```python
from build123d import *

# Parameters (mm, degrees)
SKETCH1_W           = 45
SKETCH1_H           = 57
BOSS_EXTRUDE1_DEPTH = 10
SKETCH4_W           = 45
SKETCH4_H           = 10
BOSS_EXTRUDE4_DEPTH = 35
SKETCH5_W           = 5
SKETCH5_H           = 20
SKETCH5_W_2         = 2
BOSS_EXTRUDE5_DEPTH = 45
CUT_EXTRUDE1_START  = -30
SKETCH6_R           = 1.75
CUT_EXTRUDE1_DEPTH  = 30


with BuildPart() as part:
    # Sketch1 → Boss-Extrude1 (new body)
    with BuildSketch(Plane(origin=(0, 0, 0), x_dir=(1, 0, 0), z_dir=(0, 1, 0))):
        Rectangle(SKETCH1_W, SKETCH1_H)
        with BuildLine():
            ThreePointArc((-15, -19.5), (-18, -16.5), (-15, -13.5))
            Line((-15, -13.5), (15, -13.5))
            ThreePointArc((15, -13.5), (17.121320344, -14.378679656), (18, -16.5))
            ThreePointArc((18, -16.5), (17.121320344, -18.621320344), (15, -19.5))
            Line((15, -19.5), (-15, -19.5))
        make_face(mode=Mode.SUBTRACT)
    extrude(amount=BOSS_EXTRUDE1_DEPTH)

    # Sketch4 → Boss-Extrude4 (add)
    with BuildSketch(Plane(origin=(0, 0, -28.5), x_dir=(-1, 0, 0), z_dir=(0, 0, -1))):
        with Locations((0, 5)):
            Rectangle(SKETCH4_W, SKETCH4_H)
    extrude(amount=BOSS_EXTRUDE4_DEPTH)

    # Sketch5 → Boss-Extrude5 (add)
    with BuildSketch(Plane(origin=(22.5, 0, 0), x_dir=(0, 0, -1), z_dir=(1, 0, 0))):
        with Locations((36, 20)):
            Rectangle(SKETCH5_W, SKETCH5_H)
        with Locations((48.5, 20)):
            Rectangle(SKETCH5_W_2, SKETCH5_H)
        with Locations((61, 20)):
            Rectangle(SKETCH5_W, SKETCH5_H)
    extrude(amount=-BOSS_EXTRUDE5_DEPTH)

    # Sketch6 → Cut-Extrude1 (cut)
    with BuildSketch(Plane.XY.offset(-33.5).offset(CUT_EXTRUDE1_START)):
        with Locations((0, 20)):
            Circle(SKETCH6_R)
    extrude(amount=CUT_EXTRUDE1_DEPTH, mode=Mode.SUBTRACT)


solid = part.part
```
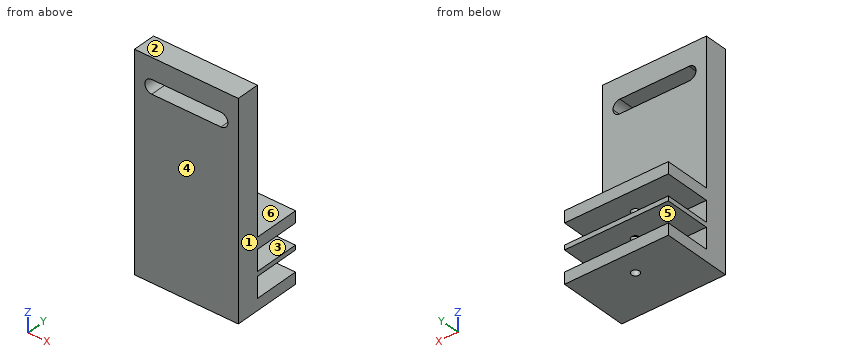
The listing builds one solid part. Answer for the finished solid, in the listing's coordinates (mm). Face numbers are marked on the shaded views. A direction names the side the tool comes from. Give positions to 0.01 mm unless a question says otherwise; leave off trailing zeros. Order: outer loops, then holes, each group sorted by start corner. A loop starts at its lowest first (then second) coordinate and runs counter-clockwise, first axis right, second up.
Item 1: Which of the six approach directions +Z, -Z, +X, -X, +Y, -Y give full straight-line access (tool end or side, diameter ignored) to the marked faces 4, 5 and 6?
From the geometry:
face 4: +Z, -Z, +X, -X, -Y
face 5: +X, -X, +Y
face 6: +Z, +X, -X, +Y
Item 2: The part is cut by section A-A, the plane y = 3.25. Give the vertices of the cut face in (x, z).
From the geometry:
outline: (-22.5, -63.5) - (22.5, -63.5) - (22.5, 28.5) - (-22.5, 28.5) - close; hole (-15, 13.5) - (15, 13.5) arc R3 ccw to (15, 19.5) - (-15, 19.5) arc R3 ccw to start
Item 3: The part is cut by section D-D, the plane y = 20. Give the vertices of the cut face in (x, z), and give its area (3 significant figures).
From the geometry:
outline: (-22.5, -63.5) - (-1.75, -63.5) - (-1.75, -58.5) - (-22.5, -58.5) - close; (-22.5, -49.5) - (-1.75, -49.5) - (-1.75, -47.5) - (-22.5, -47.5) - close; (-22.5, -38.5) - (-1.75, -38.5) - (-1.75, -33.5) - (-22.5, -33.5) - close; (1.75, -63.5) - (22.5, -63.5) - (22.5, -58.5) - (1.75, -58.5) - close; (1.75, -49.5) - (22.5, -49.5) - (22.5, -47.5) - (1.75, -47.5) - close; (1.75, -38.5) - (22.5, -38.5) - (22.5, -33.5) - (1.75, -33.5) - close
area: 498 mm2
Item 4: Find the intervals of material crossed by probe 1 along Z at (x, y) = (-10, 13.75); probe 2 along X at (y, z) = (20.25, -38); probe 3 along Z at (x, y) = (-14, 8), in increasing order.
From the geometry:
probe 1: z = -63.5 to -58.5, -49.5 to -47.5, -38.5 to -33.5
probe 2: x = -22.5 to -1.73, 1.73 to 22.5
probe 3: z = -63.5 to 13.5, 19.5 to 28.5
Item 5: The part is cut by section B-B, the plane x = -7.5. Give the vertices of the cut face in (y, z), and give its area (3 significant figures).
From the geometry:
outline: (0, -63.5) - (30, -63.5) - (30, -58.5) - (10, -58.5) - (10, -49.5) - (30, -49.5) - (30, -47.5) - (10, -47.5) - (10, -38.5) - (30, -38.5) - (30, -33.5) - (10, -33.5) - (10, 13.5) - (0, 13.5) - close; (0, 19.5) - (10, 19.5) - (10, 28.5) - (0, 28.5) - close
area: 1,100 mm2
Item 6: Given pin 1 Ø4.5 at (x, z) = (-7.5, -45) entering from +Y; pin 2 Ø6 at (x, y) = (-7.5, 22) entering from +Z, each flat-ended and moving along its own axis, determine where each tip first touches the part or whether it passes through.
From the geometry:
pin 1: stops at y = 10
pin 2: stops at z = -33.5
Item 7: The part is cut by section C-C, the plane x = 0. Count the separate pieces of the cut face and the enclosed holes in it, and give its area (3 significant figures).
From the geometry:
separate pieces: 5
enclosed holes: 0
area: 1,060 mm2
Item 8: For a pull along Z with two mould halves and no side action, classify the marked faces 1, 2 and 3 as pulls with the +Z half, pulls with the -Z half, needs draft (parallel to the pull), parting line crosses it, or undercut.
From the geometry:
face 1: needs draft
face 2: pulls with the +Z half
face 3: undercut
